Read the model definition and answer for the solid it produces. Units are mm, in the model's axes. A direction names the side the tool comes from. Give positions to 0.01 mm unless a question says otherwise; leave off trailing zeros. Loops run counter-clockwise (first coordinate to the right, second up) from the corner with the lowest first, then second, coordinate; pieces in that order, holes last. Notation, with made-up numbers: (0.25, 10.5) - (52.25, 10.5) arc R13 ccw to (52.25, 34.5) - close; hole circle Ø6 at (44, 59). An arc over 180 degrees is marked (long way). Use a Markdown table: item, result. Add a question column.
Item 1: A cutting plane is placed at D-D (x = 5.1). Determine the outline of the cut face in (y, z), plus the area to 3 significant figures.
Item 2: Each of these flat-tipped pins is pushed along its axis until it touches: P1, Ø0.5, axis at x = 5.5, z = -1.5, coming from the +Y side; P2, Ø2.5, axis at x = 4.5, y = 12.5, coming from the +Z side; P3, Ø3, axis at x = 5, z = -4.5, coming from the -Y side; P4, Ø1.6, axis at x = 4.5, z = -5, coming from the +Y side. Where does it stop, or does it pass through?
Item 3: Consider probe 1 along Z at (x, y) = (4.5, 11.3); probe 2 along Z at (x, y) = (7.1, 13.5); probe 3 along Z at (x, y) = (4.7, 12.75). Determine where each line is inside the solid, lowest interval first. Write a range as [from, to].
Item 4: For a pull along Z with two mould halves and no side action, classify faces 1 (the face through (6.6, 7.58, 9.64)), 2 (the face through (5, 11, 2)), 3 (the face through (5, 10.598, -3)) as +Z half, -Z half, draft (parallel to the pull), parting line (faces both ways), or undercut.
Item 5: A cutting plane is placed at A-A (y = 14.25). Determine the outline of the cut face in (x, z), plus the area to 3 significant figures.
Item 6: A cutting plane is placed at C-C (z = 8.5). Determine the outline of the cut face in (x, y), plus the area to 3 significant figures.
Item 7: Which of the six approach directions +Z, -Z, +X, -X, +Y, -Y give full straight-line access (tool end or side, diameter ignored) to faces 4 (the face through (4.5, 16.5, 0.1)), 5 (the face through (4, 8.598, 7)), 6 (the face through (4.542, 12.436, -1.907)), 7 (the face through (5, 13, 1))?
from build123d import *

# Parameters (mm, degrees)
BOSS_EXTRUDE1_DEPTH   = 6
SKETCH3_W             = 7.6
SKETCH3_H             = 8.4
SKETCH3_H_2           = 4.9
CUT_EXTRUDE2_DEPTH    = 21.860671783
SKETCH4_W             = 7.6
SKETCH4_H             = 3.5
SKETCH4_W_2           = 5.5
SKETCH4_H_2           = 3.1
CUT_EXTRUDE3_DEPTH    = 21.860671783
FILLET2_R             = 3
F_2_56_TAPPED_HOLE1_D = 1.778
FILLET3_R             = 0.5
F_2_56_TAPPED_HOLE2_D = 1.778
SKETCH19_R            = 0.5
CUT_EXTRUDE6_DEPTH    = 21.860671783


with BuildPart() as part:
    # Sketch1 → Boss-Extrude1 (new body)
    with BuildSketch(Plane(origin=(7.5, 0, 0), x_dir=(0, 0, -1), z_dir=(1, 0, 0))):
        with BuildLine():
            Line((-10.5, 16.997577099), (-10.5, 6.597577099))
            Line((-10.5, 6.597577099), (-2, 6.597577099))
            Line((-2, 6.597577099), (-2, 15.497577099))
            ThreePointArc((-2, 15.497577099), (-1.5, 15.997577099), (-1, 15.497577099))
            Line((-1, 15.497577099), (-1, 10.597577099))
            Line((-1, 10.597577099), (7, 10.597577099))
            Line((7, 10.597577099), (7, 16.997577099))
            Line((7, 16.997577099), (-10.5, 16.997577099))
        make_face()
    extrude(amount=-BOSS_EXTRUDE1_DEPTH)

    # Sketch3 → Cut-Extrude2 (cut, through all)
    with BuildSketch(Plane.ZY.offset(-1.5)):
        with Locations((6.7, 16.297577099)):
            Rectangle(SKETCH3_W, SKETCH3_H)
        with Locations((-3.7, 18.047577099)):
            Rectangle(SKETCH3_W, SKETCH3_H_2)
    extrude(amount=-CUT_EXTRUDE2_DEPTH, mode=Mode.SUBTRACT)

    # Sketch4 → Cut-Extrude3 (cut, through all)
    with BuildSketch(Plane.ZY.offset(-1.5)):
        with Locations((6.7, 10.347577099)):
            Rectangle(SKETCH4_W, SKETCH4_H)
        with Locations((-4.736302331, 14.047577099)):
            Rectangle(SKETCH4_W_2, SKETCH4_H_2)
    extrude(amount=-CUT_EXTRUDE3_DEPTH, mode=Mode.SUBTRACT)

    # Fillet2
    fillet2_edges = [part.edges().sort_by_distance(p)[0] for p in [
        (1.5, 7.597577099, 10.5),
        (7.5, 7.597577099, 10.5),
        (7.5, 11.547577099, -7),
        (1.5, 11.547577099, -7),
    ]]
    fillet(fillet2_edges, radius=FILLET2_R - 0.0001)  # a hair under: the kernel refuses the full size

    # #2-56 Tapped Hole1 (through all)
    with Locations(Plane(origin=(0, 8.597577099, 0), x_dir=(1, 0, 0), z_dir=(0, 1, 0))):
        with Locations((4.5, -8)):
            Hole(F_2_56_TAPPED_HOLE1_D / 2)

    # Fillet3
    fillet3_edges = [part.edges().sort_by_distance(p)[0] for p in [
        (4.5, 15.597577099, 0.1),
        (4.5, 8.597577099, 2.9),
    ]]
    fillet(fillet3_edges, radius=FILLET3_R)

    # #2-56 Tapped Hole2 (through all)
    with Locations(Plane(origin=(0, 12.497577099, 0), x_dir=(1, 0, 0), z_dir=(0, 1, 0))):
        with Locations((4.5, 5)):
            Hole(F_2_56_TAPPED_HOLE2_D / 2)

    # Sketch19 → Cut-Extrude6 (cut, through all)
    with BuildSketch(Plane(origin=(7.5, 0, 0), x_dir=(0, 0, -1), z_dir=(1, 0, 0))):
        with Locations((2.269145043, 12.780419811)):
            Circle(SKETCH19_R)
    extrude(amount=-CUT_EXTRUDE6_DEPTH, mode=Mode.SUBTRACT)


solid = part.part
Geometry says:
| question | item | result |
|---|---|---|
| 1 | outline | (6.6, 2) - (15.5, 2) arc R0.5 cw to (15.5, 1) - (10.6, 1) - (10.6, -4.34) - (12.5, -4.34) - (12.5, -2.68) arc R0.5 cw (long way) to (13.19, -1.99) - (15.6, -1.99) - (15.6, -0.4) arc R0.5 cw to (16.1, 0.1) - (17, 0.1) - (17, 2.9) - (9.1, 2.9) arc R0.5 cw to (8.6, 3.4) - (8.6, 7.34) - (6.6, 7.34) - close; (6.6, 8.66) - (8.6, 8.66) - (8.6, 10.44) - (6.6, 10.44) - close; (10.6, -6.94) - (12.5, -6.94) - (12.5, -5.66) - (10.6, -5.66) - close |
| 1 | area | 45.9 mm² |
| 2 | P1 | y = 15.6 |
| 2 | P2 | z = 2.9 |
| 2 | P3 | y = 10.6 |
| 2 | P4 | through |
| 3 | probe 1 | [-7, -5.89], [-4.11, 1], [2, 2.9] |
| 3 | probe 2 | [-1.99, 1], [2, 2.9] |
| 3 | probe 3 | [-1.77, 1], [2, 2.9] |
| 4 | face 1 | +Z half |
| 4 | face 2 | undercut |
| 4 | face 3 | draft |
| 5 | outline | (1.5, -1.99) - (7.5, -1.99) - (7.5, 1) - (1.5, 1) - close; (1.5, 2) - (7.5, 2) - (7.5, 2.9) - (1.5, 2.9) - close |
| 5 | area | 23.3 mm² |
| 6 | outline | (1.67, 6.6) - (3.76, 6.6) - (3.76, 8.6) - (1.67, 8.6) - close; (5.24, 6.6) - (7.33, 6.6) - (7.33, 8.6) - (5.24, 8.6) - close |
| 6 | area | 8.37 mm² |
| 7 | face 4 | -Z, +X, -X, +Y |
| 7 | face 5 | +Z, +X, -X, +Y |
| 7 | face 6 | +X, -X |
| 7 | face 7 | +X, -X, -Y |
